Model file for the job. Use its own axes, mm. A direction names the side the tool comes from. Coordinates: 2 decimals unless noted, no trailing zeros. Order: outer loops, then holes, each group sorted by start corner. A loop starts at its lowest first (then second) coordinate and runs counter-clockwise, first axis right, second up. Notation, with made-up numbers: (-19, 72) -> (-2, 72) arc R32 ccw to (-2, 107) -> close; hole circle Ø9 at (71, 42). An arc over 180 degrees is marked (long way). Return JSON: item names as keys, results as strings. Group by question number.
1) Cut at C-C (y = 15). Write the cut outline in (x, z).
2) Flat gauge pins, fed straight in: pin 1 (3.5 mm diameter, centred on x = 25.4, z = -6.12, fed in from -Y); pin 2 (1.4 mm diameter, centred on x = -3.5, z = -5.5, fed in from +Y); pin 3 (2 mm diameter, centred on x = 1.5, z = -6.5, fed in from -Y); pin 4 (3 mm diameter, centred on y = 3.5, z = -3.5, fed in from +X). Where does each tip first touch, or does it go through?
3) Cut at B-B (x = 12.25). Write the cut outline in (y, z) (3 decimals), and give its area (3 significant figures).
4) Which spindle directions (+Z, -Z, +X, -X, +Y, -Y) get a long thin tool onto all of the face, cutting with end or side? Do faces 4 (the flat face through (27, 17, -6.725)), 5 (the flat face through (-1, 15.76, -6)), 6 (the flat face through (9, 26.58, -6)). Say none if no direction does.
5) Pull direction Z, two halves, no side cores. Call faces 1 (the cylindrical face through (0, 25, -6)), 2 (the flat face through (16, 22.48, -6)), 3 (the cylindrical face through (24.336, 16.967, -6.163)): +Z half, -Z half, draft (parallel to the pull), parting line (faces both ways), or undercut.
6) Probe line 1 (X direction, y = 20, z = -7.5); line 2 (Y direction, x = 2, z = -10.75); line 3 (Y direction, x = 5.5, z = -2.75). List the from-to ranges inside material, lowest first.
7) Cut at D-D (z = -9.5). Write the cut outline in (x, y), and give its area (3 significant figures).
Autodesk Inventor part; units mm, degrees
ref_plane "YZ Plane" through (0, 0, 0) normal (1, 0, 0) x (0, 1, 0)
ref_plane "XZ Plane" through (0, 0, 0) normal (0, 1, 0) x (-1, 0, 0)
ref_plane "XY Plane" through (0, 0, 0) normal (0, 0, 1) x (1, 0, 0)
sketch "Sketch1" plane through (0, 0, 0) normal (0, 1, 0) x (-1, 0, 0)
  line L0 (0, 0) -> (-22.66, 0)
  line L1 (-22.66, 0) -> (-22.66, -12.25)
  line L2 (-22.66, -12.25) -> (0, -12.25)
  line L3 (0, -12.25) -> (0, 0)
  dimension "innerLength" = 22.66
  dimension "width" = 12.25
extrude "Extrusion1" add sketch "Sketch1" along normal blind 22.48
sketch "Sketch2" plane through (0, 0, -12.25) normal (-1, 0, 0) x (0, 0, 1)
  line L0 (0, 0) -> (0, 22.48)
  line L1 (0, 18.14) -> (12.25, 18.14)
  line L2 (12.25, 18.14) -> (12.25, 15.76)
  line L3 (12.25, 15.76) -> (0, 15.76)
  line L4 (0, 15.76) -> (0, 18.14)
  line L5 (0, 22.48) -> (12.25, 22.48)
  line L6 (12.25, 0) -> (12.25, 22.48)
  dimension "lipOffsetFromTop" = 4.34
  dimension "lipHeight" = 2.38
extrude "Extrusion2" add sketch "Sketch2" along normal blind 4.82 contours L0 L1 L2 L3
sketch "Sketch3" plane through (22.66, 0, 0) normal (1, 0, 0) x (0, 0, -1)
  line L0 (0, 18.14) -> (12.25, 18.14)
  line L1 (12.25, 18.14) -> (12.25, 15.76)
  line L2 (12.25, 15.76) -> (0, 15.76)
  line L3 (0, 15.76) -> (0, 18.14)
  line L4 (12.25, 0) -> (12.25, 22.48)
  line L5 (0, 0) -> (0, 22.48)
  line L6 (0, 22.48) -> (12.25, 22.48)
  dimension "d8" = 4.34
  dimension "d9" = 2.38
extrude "Extrusion3" add sketch "Sketch3" along normal blind 4.82 contours L0 L1 L2 L3
sketch "Sketch4" plane through (0, 22.48, 0) normal (0, 1, 0) x (1, 0, 0)
  arc A0 (11.646, 8.7771) -> (11.646, 3.4729) centre (6.125, 6.125) ccw
  arc A1 (11.646, 3.4729) -> (11.646, 8.7771) centre (12.25, 6.125) ccw
  line L0 (22.66, 12.25) -> (0, 12.25)
  line L1 (0, 12.25) -> (0, 0)
  line L2 (0, 0) -> (22.66, 0)
  dimension "d12" = 5.44
extrude "Extrusion4" add sketch "Sketch4" along normal blind 4.1 contours A1 A0
sketch "Sketch5" plane through (0, 26.58, 0) normal (0, 1, 0) x (1, 0, 0)
  circle A0 centre (6.125, 6.125) radius 2.435
  arc A1 (11.646, 8.7771) -> (11.646, 3.4729) centre (6.125, 6.125) ccw
  point P0 (0, 0)
  dimension "shaftDiameter" = 4.87
extrude "Extrusion5" add sketch "Sketch5" along normal blind 2.94
sketch "Sketch6" plane through (22.66, 18.14, 0) normal (0, 1, 0) x (1, 0, 0)
  arc A0 (3.62, 6.725) -> (3.62, 5.525) centre (2.7401, 6.125) ccw
  line L0 (4.82, 0) -> (4.82, 12.25)
  line L1 (4.82, 5.525) -> (3.62, 5.525)
  line L2 (4.82, 6.725) -> (3.62, 6.725)
  line L3 (0, 12.25) -> (4.82, 12.25)
  point P0 (-22.66, 0)
  dimension "mountingHoleDiameter" = 2.13
  dimension "d19" = 1.2
  dimension "d20" = 1.2
  dimension "d21" = 0.6
  dimension "d22" = 6.125
  dimension "mountingHoleOffset" = 2.0799
extrude "Extrusion6" cut sketch "Sketch6" against normal through all
sketch "Sketch7" plane through (0, 18.14, 0) normal (0, 1, 0) x (1, 0, 0)
  arc A0 (-3.62, 5.525) -> (-3.62, 6.725) centre (-2.7401, 6.125) ccw
  line L0 (0, 12.25) -> (-4.82, 12.25)
  line L1 (-4.82, 5.525) -> (-3.62, 5.525)
  line L2 (-4.82, 6.725) -> (-3.62, 6.725)
  line L3 (-4.82, 0) -> (-4.82, 12.25)
  line L4 (-4.82, 6.725) -> (-4.82, 5.525)
  point P0 (0, 0)
  dimension "d27" = 2.13
  dimension "d29" = 6.125
  dimension "d31" = 1.2
  dimension "d32" = 1.2
  dimension "d33" = 0.6
extrude "Extrusion7" cut sketch "Sketch7" against normal through all
sketch "Sketch8" plane through (0, 0, -12.25) normal (-1, 0, 0) x (0, 0, 1)
  circle A0 centre (5.125, 5) radius 0.5
  circle A1 centre (6.125, 5) radius 0.5
  circle A2 centre (7.125, 5) radius 0.5
  line L0 (0, 0) -> (0, 15.76)
  line L1 (2.9548, 5) -> (8.7957, 5)
  line L2 (0, 0) -> (12.25, 0)
  dimension "d36" = 1
  dimension "d37" = 6.125
  dimension "d38" = 5
extrude "Extrusion8" add sketch "Sketch8" along normal blind 2
equation "\"lipLength\" = -0.5 * innerLength + 0.5 * length"
equation "\"d8\" = lipOffsetFromTop"
equation "\"d9\" = lipHeight"
equation "\"d10\" = lipLength"
equation "\"d20\" = d19"
equation "\"d21\" = 0.5 * d19"
equation "\"d22\" = 0.5 * width"
equation "\"d27\" = mountingHoleDiameter"
equation "\"d29\" = 0.5 * width"
equation "\"d31\" = d19"
equation "\"d32\" = d19"
equation "\"d33\" = 0.5 * d19"
equation "\"d37\" = 0.5 * width"
equation "\"length\" = 32.3"
properties part number "micro-servo"
Answers below:
{
 "1": {"outline": "(0, -12.25) -> (22.66, -12.25) -> (22.66, 0) -> (0, 0) -> close"},
 "2": {"pin 1": "stops at y = 15.76", "pin 2": "stops at y = 18.14", "pin 3": "stops at y = 0", "pin 4": "stops at x = 22.66"},
 "3": {"outline": "(0, -12.25) -> (22.48, -12.25) -> (22.48, -8.845) -> (26.58, -8.845) -> (26.58, -3.405) -> (22.48, -3.405) -> (22.48, 0) -> (0, 0) -> close", "area": "298 mm^2"},
 "4": {"face 4": "+X, +Y, -Y", "face 5": "+Z, -Z, -X", "face 6": "+Y"},
 "5": {"face 1": "parting line", "face 2": "draft", "face 3": "undercut"},
 "6": {"line 1": "x = 0 to 22.66", "line 2": "y = 0 to 22.48", "line 3": "y = 0 to 26.58"},
 "7": {"outline": "(-4.82, 15.76) -> (0, 15.76) -> (0, 0) -> (22.66, 0) -> (22.66, 15.76) -> (27.48, 15.76) -> (27.48, 18.14) -> (22.66, 18.14) -> (22.66, 22.48) -> (11.24, 22.48) -> (11.24, 26.58) -> (1.01, 26.58) -> (1.01, 22.48) -> (0, 22.48) -> (0, 18.14) -> (-4.82, 18.14) -> close", "area": "574 mm^2"}
}
